```python
from build123d import *

# Parameters (mm, degrees)
BOSS_EXTRUDE1_DEPTH = 5
BOSS_EXTRUDE2_DEPTH = 10
BOSS_EXTRUDE3_DEPTH = 3
BOSS_EXTRUDE4_DEPTH = 5
FILLET1_R           = 10


with BuildPart() as part:
    # Sketch1 → Boss-Extrude1 (new body)
    with BuildSketch(Plane.XY):
        Polygon((-150, 75.248916092), (0, 0), (150, 75.248916092), (150, 52.873374138), (22.301525839, -11.187770977), (119.603051678, -60), (75, -60), (0, -22.375541954), (-75, -60), (-119.603051678, -60), (-22.301525839, -11.187770977), (-150, 52.873374138), align=None)
    extrude(amount=BOSS_EXTRUDE1_DEPTH)

    # Sketch2 → Boss-Extrude2 (add)
    with BuildSketch(Plane.XY.offset(5)):
        Polygon((-150, 75.248916092), (-150, 52.873374138), (-147, 51.368395816), (-147, 73.74393777), align=None)
        Polygon((150, 75.248916092), (147, 73.74393777), (147, 51.368395816), (150, 52.873374138), align=None)
        Polygon((119.603051678, -60), (111.629514899, -56), (67.026463221, -56), (75, -60), align=None)
        Polygon((-75, -60), (-119.603051678, -60), (-111.629514899, -56), (-67.026463221, -56), align=None)
    extrude(amount=BOSS_EXTRUDE2_DEPTH)

    # Sketch3 → Boss-Extrude3 (add)
    with BuildSketch(Plane.XY.offset(15)):
        Polygon((-150, 75.248916092), (-150, 52.873374138), (-140, 47.856779731), (-140, 70.232321686), align=None)
        Polygon((-75, -60), (-55.066158054, -50), (-99.669209731, -50), (-119.603051678, -60), align=None)
        Polygon((75, -60), (119.603051678, -60), (99.669209731, -50), (55.066158054, -50), align=None)
        Polygon((150, 75.248916092), (140, 70.232321686), (140, 47.856779731), (150, 52.873374138), align=None)
    extrude(amount=BOSS_EXTRUDE3_DEPTH)

    # Sketch4 → Boss-Extrude4 (add)
    with BuildSketch(Plane.XY):
        with BuildLine():
            Line((-62.568316909, 31.387986861), (0, 0))
            Line((0, 0), (62.568316909, 31.387986861))
            ThreePointArc((62.568316909, 31.387986861), (0, 70), (-62.568316909, 31.387986861))
        make_face()
    extrude(amount=BOSS_EXTRUDE4_DEPTH)

    # Fillet1
    fillet1_edges = [part.edges().sort_by_distance(p)[0] for p in [
        (62.568316909, 31.387986861, 2.5),
        (-62.568316909, 31.387986861, 2.5),
    ]]
    fillet(fillet1_edges, radius=FILLET1_R)


solid = part.part
```
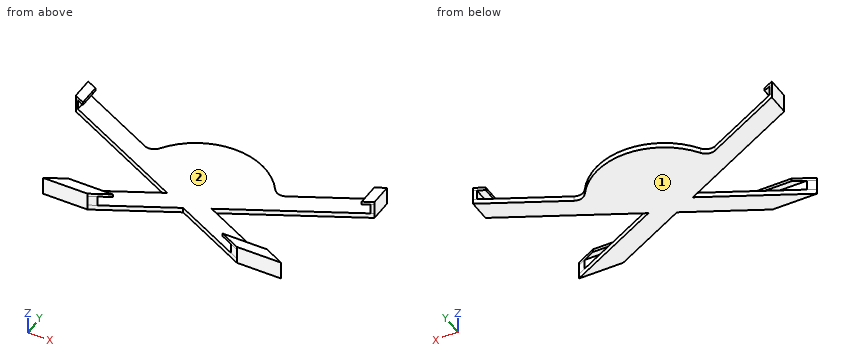
The model under review builds one solid part; all positions refer to its coordinate system, in mm. Face numbers are marked on the shaded views. Coordinates: 2 decimals unless noted, no trailing zeros. Write each loop counter-clockwise with the first axis right and the second up, starting at its lowest first coordinate (ties: lowest second). Pieces come first, ordered by that corner, then holes.
1) We need section A-A on z = 9.75. State the section outline as (x, y) points.
2) We need section D-D on y = 64.5. State the section outline as (x, z) points, then the cut area to 3 significant figures.
3) To check wall thickness, follow probe 1 along Z at (x, y) = (128, 42); probe 2 along Y at (x, z) = (100, 6); probe 3 along Y at (x, z) = (30, 3.75). State the ranges of each line that lie inside material, in increasing order.
4) Clearance check with flat-ended pins moving along their axes: pin 1 Ø6 at (x, y) = (-45.5, 31.5) entering from -Z; pin 2 Ø2.5 at (x, z) = (69, 17) entering from +Y; pin 3 Ø2 at (x, z) = (-118.5, 13) entering from +Y (3 decimals); pin 4 Ø8 at (x, z) = (22, 4.5) entering from -Y. State where each tip first meets the part, or that it passes through.
5) We need section B-B on x = -85.5. State the section outline as (y, z) points.
6) We need section C-C on y = -34.5. State the section outline as (x, z) points, then the cut area to 3 significant figures.
7) The part is to be moulded in two halves that separate along X. For the marked faces 1 and 2, say which applies: pulls with the +X half, pulls with the -X half, needs draft (parallel to the pull), parting line crosses it, or undercut.
Answer list:
1. outline: (-150, 52.87) - (-147, 51.37) - (-147, 73.74) - (-150, 75.25) - close; (-119.6, -60) - (-75, -60) - (-67.03, -56) - (-111.63, -56) - close; (67.03, -56) - (75, -60) - (119.6, -60) - (111.63, -56) - close; (147, 51.37) - (150, 52.87) - (150, 75.25) - (147, 73.74) - close
2. outline: (-150, 0) - (-128.57, 0) - (-128.57, 5) - (-147, 5) - (-147, 15) - (-140, 15) - (-140, 18) - (-150, 18) - close; (-27.2, 0) - (27.2, 0) - (27.2, 5) - (-27.2, 5) - close; (128.57, 0) - (150, 0) - (150, 18) - (140, 18) - (140, 15) - (147, 15) - (147, 5) - (128.57, 5) - close
2. area: 606 mm2
3. probe 1: z = 0 to 5
3. probe 2: y = -60 to -56
3. probe 3: y = -37.43 to -15.05, -7.33 to 63.25
4. pin 1: stops at z = 0
4. pin 2: stops at y = -50
4. pin 3: stops at y = -58.945
4. pin 4: stops at y = -35.42
5. outline: (-60, 0) - (-42.89, 0) - (-42.89, 5) - (-56, 5) - (-56, 15) - (-50, 15) - (-50, 18) - (-60, 18) - close; (20.52, 0) - (42.89, 0) - (42.89, 5) - (20.52, 5) - close
6. outline: (-68.77, 0) - (-24.17, 0) - (-24.17, 5) - (-68.77, 5) - close; (24.17, 0) - (68.77, 0) - (68.77, 5) - (24.17, 5) - close
6. area: 446 mm2
7. face 1: needs draft
7. face 2: undercut
